Verification items for the finished model (mm, model axes). A direction names the side the tool comes from. Give positions to 0.01 mm unless a question says otherwise; leave off trailing zeros. Loops run counter-clockwise (first coordinate to the right, second up) from the corner with the lowest first, then second, coordinate; pieces in that order, holes last. Notation, with made-up numbers: M -38.75,63 L -2.75,63 A21 ccw -2.75,78 Z; hole C 35,88.5 d4. An arc over 180 degrees is marked long. Answer in a Markdown table with one row per item.
```python
from build123d import *

# Parameters (mm, degrees)
SKETCH1_W            = 102
SKETCH1_H            = 18
BOSS_EXTRUDE1_DEPTH  = 2
BOSS_EXTRUDE2_DEPTH  = 18
SKETCH4_W            = 81
SKETCH4_H            = 2
BOSS_EXTRUDE3_DEPTH  = 6
SKETCH5_W            = 2.3
SKETCH5_H            = 2
CUT_EXTRUDE1_DEPTH   = 6
SKETCH8_W            = 2
SKETCH8_H            = 6
BOSS_EXTRUDE5_DEPTH  = 1
SKETCH10_W           = 3.5
SKETCH10_H           = 6
BOSS_EXTRUDE6_DEPTH  = 1
SKETCH11_W           = 1.5
SKETCH11_H           = 6
BOSS_EXTRUDE7_DEPTH  = 8
BOSS_EXTRUDE8_DEPTH  = 6
RIB1_REACH           = 54.402
SKETCH17_WALL_W      = 117.434725866
SKETCH17_WALL_H      = 4
CHAMFER1_SIZE        = 0.5
SKETCH18_W           = 7.5
SKETCH18_H           = 3.4
BOSS_EXTRUDE10_DEPTH = 4
SKETCH19_W           = 26.1754507
SKETCH19_H           = 11
CUT_EXTRUDE3_DEPTH   = 1
SKETCH20_W           = 2.3
SKETCH20_H           = 1
CUT_EXTRUDE4_DEPTH   = 18


with BuildPart() as part:
    # Sketch1 → Boss-Extrude1 (new body)
    with BuildSketch(Plane.XY):
        Rectangle(SKETCH1_W, SKETCH1_H)
    extrude(amount=BOSS_EXTRUDE1_DEPTH)

    # Sketch2 → Boss-Extrude2 (add)
    with BuildSketch(Plane(origin=(0, 9, 0), x_dir=(1, 0, 0), z_dir=(0, 1, 0))):
        Polygon((-43.5, 0), (-40.5, 0), (-40.5, 6), (-51, 6), (-51, 3.4), (-43.5, 3.4), align=None)
        Polygon((40.5, 6), (40.5, 0), (43.5, 0), (43.5, 3.4), (51, 3.4), (51, 6), align=None)
    extrude(amount=-BOSS_EXTRUDE2_DEPTH)

    # Sketch4 → Boss-Extrude3 (add)
    with BuildSketch(Plane(origin=(0, 0, 0), x_dir=(-1, 0, 0), z_dir=(0, 0, -1))):
        with Locations((0, 8)):
            Rectangle(SKETCH4_W, SKETCH4_H)
        with Locations((0, -8)):
            Rectangle(SKETCH4_W, SKETCH4_H)
    extrude(amount=BOSS_EXTRUDE3_DEPTH)

    # Sketch5 → Cut-Extrude1 (cut)
    with BuildSketch(Plane(origin=(0, 0, -6), x_dir=(-1, 0, 0), z_dir=(0, 0, -1))):
        with Locations((26.75, -8)):
            Rectangle(SKETCH5_W, SKETCH5_H)
        with Locations((26.75, 8)):
            Rectangle(SKETCH5_W, SKETCH5_H)
        with Locations((-20.25, 8)):
            Rectangle(SKETCH5_W, SKETCH5_H)
        with Locations((-20.25, -8)):
            Rectangle(SKETCH5_W, SKETCH5_H)
    extrude(amount=-CUT_EXTRUDE1_DEPTH, mode=Mode.SUBTRACT)

    # Sketch8 → Boss-Extrude5 (add)
    with BuildSketch(Plane(origin=(0, 0, 0), x_dir=(-1, 0, 0), z_dir=(0, 0, -1))):
        with Locations((33.75, 0)):
            Rectangle(SKETCH8_W, SKETCH8_H)
        with Locations((-13.25, 0)):
            Rectangle(SKETCH8_W, SKETCH8_H)
    extrude(amount=BOSS_EXTRUDE5_DEPTH)

    # Sketch10 → Boss-Extrude6 (add)
    with BuildSketch(Plane(origin=(0, 0, -1), x_dir=(-1, 0, 0), z_dir=(0, 0, -1))):
        with Locations((-14, 0)):
            Rectangle(SKETCH10_W, SKETCH10_H)
        with Locations((33, 0)):
            Rectangle(SKETCH10_W, SKETCH10_H)
    extrude(amount=BOSS_EXTRUDE6_DEPTH)

    # Sketch11 → Boss-Extrude7 (add)
    with BuildSketch(Plane(origin=(0, 0, 0), x_dir=(-1, 0, 0), z_dir=(0, 0, -1))):
        with Locations((5.8, 0)):
            Rectangle(SKETCH11_W, SKETCH11_H)
        with Locations((-41.2, 0)):
            Rectangle(SKETCH11_W, SKETCH11_H)
    extrude(amount=BOSS_EXTRUDE7_DEPTH)

    # Sketch12 → Boss-Extrude8 (add)
    with BuildSketch(Plane.XZ.offset(3)):
        Polygon((-6.55, -8), (-7.55, -6), (-6.55, -6), align=None)
        Polygon((40.45, -8), (39.45, -6), (40.45, -6), align=None)
    extrude(amount=-BOSS_EXTRUDE8_DEPTH)

    # Sketch17 wall → Rib1 (add, up to next)
    with BuildSketch(Plane(origin=(-1.55, 0, -4), x_dir=(0.658504607869, 0, 0.752576694707), z_dir=(0.752576694707, 0, -0.658504607869)), mode=Mode.PRIVATE) as rib1_sk1:
        Rectangle(SKETCH17_WALL_W, SKETCH17_WALL_H)
    rib1_tool1 = extrude(rib1_sk1.sketch, amount=-RIB1_REACH, mode=Mode.PRIVATE) - part.part
    add(rib1_tool1.solids().sort_by_distance((-1.55, 0, -4))[0])

    # Chamfer1
    chamfer1_edges = [part.edges().sort_by_distance(p)[0] for p in [
        (-31.25, 0, -1),
        (15.75, 0, -1),
    ]]
    chamfer(chamfer1_edges, length=CHAMFER1_SIZE)

    # Sketch18 → Boss-Extrude10 (add)
    with BuildSketch(Plane.XZ.offset(9)):
        with Locations((47.25, -1.7)):
            Rectangle(SKETCH18_W, SKETCH18_H)
        with Locations((-47.25, -1.7)):
            Rectangle(SKETCH18_W, SKETCH18_H)
    extrude(amount=-BOSS_EXTRUDE10_DEPTH)

    # Sketch19 → Cut-Extrude3 (cut)
    with BuildSketch(Plane(origin=(0, 0, 0), x_dir=(-1, 0, 0), z_dir=(0, 0, -1))):
        with Locations((19.63772535, 0)):
            Rectangle(SKETCH19_W, SKETCH19_H)
        with Locations((-27.35772535, -0.484068742)):
            Rectangle(SKETCH19_W, SKETCH19_H)
    extrude(amount=-CUT_EXTRUDE3_DEPTH, mode=Mode.SUBTRACT)

    # Sketch20 → Cut-Extrude4 (cut)
    with BuildSketch(Plane(origin=(0, 9, 0), x_dir=(1, 0, 0), z_dir=(0, 1, 0))):
        with Locations((-26.75, -0.5)):
            Rectangle(SKETCH20_W, SKETCH20_H)
        with Locations((20.25, -0.5)):
            Rectangle(SKETCH20_W, SKETCH20_H)
    extrude(amount=-CUT_EXTRUDE4_DEPTH, mode=Mode.SUBTRACT)


solid = part.part
```
Item 1: Sectioned sample at B-B (z = -5). State how many separate pieces and enclosed holes the cut face has, and give its area (3 significant figures).
Reported:
| item | result |
|---|---|
| separate pieces | 5 |
| enclosed holes | 0 |
| area | 703 mm^2 |
Item 2: Scan lines: L1, parallel to X at y = 7.75, z = -3; L2, parallel to X at y = -0.25, z = -2.25; L3, parallel to X at y = 2.25, z = -1.75. Record each from-to range of solid material in increasing order. Write a range as [from, to].
Reported:
| item | result |
|---|---|
| L1 | x = [-43.5, -27.9], [-25.6, 19.1], [21.4, 43.5] |
| L2 | x = [-43.5, -40.5], [-6.55, -0.02], [40.45, 43.5] |
| L3 | x = [-43.5, -40.5], [-34.75, -31.25], [-6.55, -5.05], [12.25, 15.75], [40.45, 43.5] |
Item 3: Go/stop test with flat-tipped pins: pin 1 (1.6 mm diameter, centred on y = -0.5, z = -6.5, fed in from +X); pin 2 (1 mm diameter, centred on y = 0, z = -1, fed in from -X); pin 3 (8 mm diameter, centred on x = -46.5, y = -1, fed in from -Z). Record where each tip stops, or that it passes through.
Reported:
| item | result |
|---|---|
| pin 1 | stops at x = 51 |
| pin 2 | stops at x = -43.5 |
| pin 3 | stops at z = -6 |
Item 4: Tool access check on faces 1 (the flat face through (-3, 2, -3)), 2 (the flat face through (47, -5, -2)), 3 (the flat face through (-27.9, 8, -3)), 4 (the flat face through (-44, 0, -6)), 5 (the flat face through (-1, 0, 2)). Record the directions out of +Z, -Z, +X, -X, +Y, -Y that give a thin tool (end or side, any length) a straight path to the whole face; none if there is none.
Reported:
| item | result |
|---|---|
| face 1 | -Z |
| face 2 | +X, +Y |
| face 3 | -Z, +Y, -Y |
| face 4 | -Z, -X, +Y, -Y |
| face 5 | +Z, +X, -X, +Y, -Y |
Item 5: Sectioned sample at C-C (x = -2). Record the cut outline in (y, z), and give its area (3 significant figures).
Reported:
| item | result |
|---|---|
| outline | M -9,-6 L -7,-6 L -7,0 L -2,0 L -2,-4.51 L 2,-4.51 L 2,0 L 7,0 L 7,-6 L 9,-6 L 9,2 L -9,2 Z |
| area | 78.1 mm^2 |
Item 6: Release check for a two-part mould opening along X. For faces 6 (the flat face through (51, -2, -4)), 7 (the flat face through (-47, -5, -2)), 8 (the flat face through (12.25, 0, -1)) record: released by +X, released by -X, zero draft, split by the parting line, or undercut.
Reported:
| item | result |
|---|---|
| face 6 | released by +X |
| face 7 | zero draft |
| face 8 | undercut |
Item 7: Sectioned sample at A-A (x = -29). Record the cut outline in (y, z), and give its area (3 significant figures).
Reported:
| item | result |
|---|---|
| outline | M -9,-6 L -7,-6 L -7,0 L -5.5,0 L -5.5,1 L 5.5,1 L 5.5,0 L 7,0 L 7,-6 L 9,-6 L 9,2 L -9,2 Z |
| area | 49.0 mm^2 |
